Here's how the part is built. I have some questions about the finished solid (model axes, mm). A direction names the side the tool comes from. Round coordinates to 2 decimals unless told otherwise and drop trailing zeros. Order: outer loops, then holes, each group sorted by start corner. A loop starts at its lowest first (then second) coordinate and runs counter-clockwise, first axis right, second up. Notation, with made-up numbers: (12.5, 43.5) - (31.5, 43.5) arc R26 ccw to (31.5, 69.5) - close; hole circle Ø3 at (46, -28). An arc over 180 degrees is marked (long way). One line per item, written item: value.
from build123d import *

# Parameters (mm, degrees)
SKETCH064_W     = 35
SKETCH064_H     = 30
PAD030_DEPTH    = 14
SKETCH065_W     = 30
SKETCH065_H     = 20
POCKET041_DEPTH = 10
PAD031_DEPTH    = 4
FILLET012_R     = 6
SKETCH067_R     = 2
POCKET042_DEPTH = 4.001
CHAMFER026_SIZE = 4
CHAMFER027_SIZE = 2
CHAMFER028_SIZE = 1


with BuildPart() as part:
    # Sketch064 → Pad030 (new body)
    with BuildSketch(Plane.XY):
        with Locations((-217.5, -99)):
            Rectangle(SKETCH064_W, SKETCH064_H)
    extrude(amount=PAD030_DEPTH)

    # Sketch065 (on Face5 of Pad030) → Pocket041 (cut)
    with BuildSketch(Plane(origin=(0, 0, 0), x_dir=(1, 0, 0), z_dir=(0, 0, -1))):
        with Locations((-215, 99)):
            Rectangle(SKETCH065_W, SKETCH065_H)
    extrude(amount=-POCKET041_DEPTH, mode=Mode.SUBTRACT)

    # Sketch066 (on Face4 of Pocket041) → Pad031 (join)
    with BuildSketch(Plane(origin=(0, 0, 0), x_dir=(1, 0, 0), z_dir=(0, 0, -1))):
        Polygon((-235, 114), (-217.5, 129), (-200, 114), align=None)
        Polygon((-235, 84), (-217.5, 69), (-200, 84), align=None)
    extrude(amount=-PAD031_DEPTH)

    # Fillet012
    fillet012_edges = [part.edges().sort_by_distance(p)[0] for p in [
        (-217.5, -129, 2),
        (-217.5, -69, 2),
    ]]
    fillet(fillet012_edges, radius=FILLET012_R)

    # Sketch067 (on Face1 of Fillet012) → Pocket042 (cut, through all)
    with BuildSketch(Plane.XY.offset(4)):
        with Locations((-217.5, -76.902467)):
            Circle(SKETCH067_R)
        with Locations((-217.5, -121.097533)):
            Circle(SKETCH067_R)
    extrude(amount=-POCKET042_DEPTH, mode=Mode.SUBTRACT)

    # Chamfer026
    chamfer026_edges = [part.edges().sort_by_distance(p)[0] for p in [
        (-235, -99, 14),
        (-217.5, -114, 14),
        (-217.5, -84, 14),
    ]]
    chamfer(chamfer026_edges, length=CHAMFER026_SIZE)

    # Chamfer027
    chamfer027_edges = [part.edges().sort_by_distance(p)[0] for p in [
        (-219.5, -121.097533, 4),
        (-219.5, -76.902467, 4),
    ]]
    chamfer(chamfer027_edges, length=CHAMFER027_SIZE)

    # Chamfer028
    chamfer028_edges = [part.edges().sort_by_distance(p)[0] for p in [
        (-217.5, -127.097533, 4),
        (-217.5, -70.902467, 4),
    ]]
    chamfer(chamfer028_edges, length=CHAMFER028_SIZE)


with BuildPart() as part_1:
    # Body023 placement: moved
    add(part.part.moved(Location((0, 0, 15.5))))


solid = part_1.part
Q1. If we section it at B-B, the plane z = 21: Please give me the cut outline in (x, y), then the cut area to 3 significant figures.
Results list:
outline: (-235, -114) - (-200, -114) - (-200, -109) - (-230, -109) - (-230, -89) - (-200, -89) - (-200, -84) - (-235, -84) - close
area: 450 mm²
Q2. We'd pull the mould along Y, two halves only. Please class faces 1 (the flat face through (-218, -82, 19.5)), 2 (the flat face through (-207.214, -119.534, 18.993)), 3 (the flat face through (-230, -99, 20)): released by +Y, released by -Y, zero draft, split by the parting line, or undercut.
Results list:
face 1: zero draft
face 2: released by -Y
face 3: undercut
Q3. Which directions (+Z, -Z, +X, -X, +Y, -Y) give clear straight access to the entire face, cutting with the end or side of a thin tool? Please do faces 4 (the flat face through (-216, -99, 29.5)), 5 (the flat face through (-215, -99, 25.5)).
Results list:
face 4: +Z, +X, -X, +Y, -Y
face 5: -Z, +X
Q4. If I drill on line 1 along Y through (x, z) = (-217.5, 17.1); line 2 along X through (y, z) = (-95, 21); line 3 along X through (y, z) = (-120, 17.5), over which ranges is the centre line in solid material (lowest first)?
Results list:
line 1: -127.1 to -123.1, -119.1 to -109, -89 to -78.9, -74.9 to -70.9
line 2: -235 to -230
line 3: -228 to -219.17, -215.83 to -207
Q5. If we section it at A-A, the plane x = -217.5: Please give me the cut outline in (y, z), then the cut area to 3 significant figures.
Results list:
outline: (-127.1, 15.5) - (-123.1, 15.5) - (-123.1, 17.5) - (-125.1, 19.5) - (-126.1, 19.5) - (-127.1, 18.5) - close; (-119.1, 15.5) - (-109, 15.5) - (-109, 25.5) - (-89, 25.5) - (-89, 15.5) - (-78.9, 15.5) - (-78.9, 17.5) - (-80.9, 19.5) - (-84, 19.5) - (-84, 25.5) - (-88, 29.5) - (-110, 29.5) - (-114, 25.5) - (-114, 19.5) - (-117.1, 19.5) - (-119.1, 17.5) - close; (-74.9, 15.5) - (-70.9, 15.5) - (-70.9, 18.5) - (-71.9, 19.5) - (-72.9, 19.5) - (-74.9, 17.5) - close
area: 268 mm²
Q6. If we section it at C-C, the plane y = -103.5: Please give me the cut outline in (x, z).
Results list:
outline: (-235, 15.5) - (-230, 15.5) - (-230, 25.5) - (-200, 25.5) - (-200, 29.5) - (-231, 29.5) - (-235, 25.5) - close
Q7. Will these pins go through, and if not, where does the flat tip stop? pin 1 (8 mm diameter, centred on x = -228.5, z = 19.5, fed in from +Y); pin 2 (7.5 mm diameter, centred on x = -215, z = 23, fed in from +Y); pin 3 (1.5 mm diameter, centred on x = -204.5, z = 22, fed in from +Y).
Results list:
pin 1: y = -75.11
pin 2: y = -72.01
pin 3: y = -84
Q8. If we section it at D-D, the plane x = -205.5: Please give me the cut outline in (y, z), then the cut area to 3 significant figures.
Results list:
outline: (-118.71, 15.5) - (-109, 15.5) - (-109, 25.5) - (-89, 25.5) - (-89, 15.5) - (-79.29, 15.5) - (-79.29, 18.5) - (-80.6, 19.5) - (-84, 19.5) - (-84, 25.5) - (-88, 29.5) - (-110, 29.5) - (-114, 25.5) - (-114, 19.5) - (-117.4, 19.5) - (-118.71, 18.5) - close
area: 240 mm²
